The model under review builds one solid part; all positions refer to its coordinate system, in mm. Round coordinates to 2 decimals unless told otherwise and drop trailing zeros. Order: outer loops, then holes, each group sorted by start corner. A loop starts at its lowest first (then second) coordinate and runs counter-clockwise, first axis right, second up.
1) Mouldability with a two-part tool opening along X and no side actions: class faces 1 (the face through (38.112, 0.558, 6.261)), 2 (the face through (114.294, 0.559, 6.261)), 3 (the face through (-49, -25.4, 6)) as pulls with the +X half, pulls with the -X half, needs draft (parallel to the pull), parting line crosses it, or undercut.
2) Consider section B-B (y = 0). Give the boundary of the cut face in (x, z).
3) To check wall thickness, follow L1, parallel to Y at x = -88.9, z = 4; L2, parallel to X at y = -11, z = 10; L3, parallel to X at y = 8.5, z = 5.5. State the ranges of each line that lie inside material, in increasing order.
4) Consider section A-A (z = 4). Give the boundary of the cut face in (x, y), then the cut area to 3 significant figures.
5) Consider section D-D (x = 10.5). Give the boundary of the cut face in (y, z), then the cut area to 3 significant figures.
6) Consider section C-C (x = -88.9). Give the boundary of the cut face in (y, z).
7) Clearance check with flat-ended pins moving along their axes: P1, Ø6, axis at y = 6, z = 3, coming from the +X side; P2, Ø5, axis at y = 9, z = 6, coming from the +X side. State where each tip first meets the part, or that it passes through.
from build123d import *

# Parameters (mm, degrees)
SKETCH1_R           = 12.7
BOSS_EXTRUDE1_DEPTH = 12.7


with BuildPart() as part:
    # Sketch1 → Boss-Extrude1 (new body)
    with BuildSketch(Plane.XY):
        with BuildLine():
            Line((-88.9, 25.4), (88.9, 25.4))
            ThreePointArc((88.9, 25.4), (114.3, 0), (88.9, -25.4))
            Line((88.9, -25.4), (-88.9, -25.4))
            Line((-88.9, -25.4), (-190.5, -25.4))
            ThreePointArc((-190.5, -25.4), (-215.9, 0), (-190.5, 25.4))
            Line((-190.5, 25.4), (-88.9, 25.4))
        make_face()
        with Locations((-88.9, 0)):
            Circle(SKETCH1_R, mode=Mode.SUBTRACT)
        with Locations((88.9, 0)):
            Circle(SKETCH1_R, mode=Mode.SUBTRACT)
        with Locations((50.8, 0)):
            Circle(SKETCH1_R, mode=Mode.SUBTRACT)
        with Locations((12.7, 0)):
            Circle(SKETCH1_R, mode=Mode.SUBTRACT)
        with Locations((-25.4, 0)):
            Circle(SKETCH1_R, mode=Mode.SUBTRACT)
    extrude(amount=BOSS_EXTRUDE1_DEPTH)


solid = part.part
Answer below:
1. face 1: undercut
1. face 2: pulls with the +X half
1. face 3: needs draft
2. outline: (-215.9, 0) - (-101.6, 0) - (-101.6, 12.7) - (-215.9, 12.7) - close; (-76.2, 0) - (-38.1, 0) - (-38.1, 12.7) - (-76.2, 12.7) - close; (-12.7, 0) - (0, 0) - (0, 12.7) - (-12.7, 12.7) - close; (25.4, 0) - (38.1, 0) - (38.1, 12.7) - (25.4, 12.7) - close; (63.5, 0) - (76.2, 0) - (76.2, 12.7) - (63.5, 12.7) - close; (101.6, 0) - (114.3, 0) - (114.3, 12.7) - (101.6, 12.7) - close
3. L1: y = -25.4 to -12.7, 12.7 to 25.4
3. L2: x = -213.39 to -95.25, -82.55 to -31.75, -19.05 to 6.35, 19.05 to 44.45, 57.15 to 82.55, 95.25 to 111.79
3. L3: x = -214.44 to -98.34, -79.46 to -34.84, -15.96 to 3.26, 22.14 to 41.36, 60.24 to 79.46, 98.34 to 112.84
4. outline: (-190.5, -25.4) - (88.9, -25.4) arc R25.4 ccw to (88.9, 25.4) - (-190.5, 25.4) arc R25.4 ccw to start; hole circle Ø25.4 at (-88.9, 0); hole circle Ø25.4 at (-25.4, 0); hole circle Ø25.4 at (12.7, 0); hole circle Ø25.4 at (50.8, 0); hole circle Ø25.4 at (88.9, 0)
4. area: 13,700 mm2
5. outline: (-25.4, 0) - (-12.51, 0) - (-12.51, 12.7) - (-25.4, 12.7) - close; (12.51, 0) - (25.4, 0) - (25.4, 12.7) - (12.51, 12.7) - close
5. area: 327 mm2
6. outline: (-25.4, 0) - (-12.7, 0) - (-12.7, 12.7) - (-25.4, 12.7) - close; (12.7, 0) - (25.4, 0) - (25.4, 12.7) - (12.7, 12.7) - close
7. P1: stops at x = 114.12
7. P2: stops at x = 113.45
